Part model, mm, in its own coordinate system. Face numbers are marked on the shaded views. Give positions to 0.01 mm unless a question says otherwise; leave off trailing zeros. Order: outer loops, then holes, each group sorted by start corner. A loop starts at its lowest first (then second) coordinate and runs counter-clockwise, first axis right, second up. Notation, with made-up numbers: (56.25, 89.25) -> (87.25, 89.25) arc R22 ccw to (87.25, 118.25) -> close; hole circle Ø2 at (17.25, -30). An arc over 180 degrees is marked (long way). Write item = value, one per line. Start each with the question number.
(1) Flat gauge pins, fed straight in: pin 1 (3 mm diameter, centred on x = 4, z = 3.5, fed in from -Y); pin 2 (2 mm diameter, centred on y = -3, z = 7.5, fed in from -X); pin 3 (2 mm diameter, centred on x = 2, z = 4, fed in from -Y). Where does each tip first touch, or does it go through?
(2) Saw through at B-B, the plane x = 2.5. List the corners of the cut face in (y, z), then the cut area to 3 significant figures.
(3) Two-plate mould, pull along X, no slides. Class the marked faces 1, 2 and 3: pulls with the +X half, pulls with the -X half, needs draft (parallel to the pull), parting line crosses it, or undercut.
(4) Probe line 1 along Y through (x, z) = (0, 6.5); line 2 along Z through (x, y) = (0, 1.5); line 3 along X through (y, z) = (0.5, 4). List the from-to ranges inside material, lowest first. Write a range as from..to.
(5) Saw through at A-A, the plane y = 0. List the corners of the cut face in (x, z).
(6) Saw through at D-D, the plane y = -2. List the corners of the cut face in (x, z), then the cut area to 3 significant figures.
(7) Saw through at C-C, the plane z = 3. List the corners of the cut face in (x, y).
Autodesk Inventor part; units mm, degrees
ref_plane "YZ Plane" through (0, 0, 0) normal (1, 0, 0) x (0, 1, 0)
ref_plane "XZ Plane" through (0, 0, 0) normal (0, 1, 0) x (-1, 0, 0)
ref_plane "XY Plane" through (0, 0, 0) normal (0, 0, 1) x (1, 0, 0)
sketch "Sketch1" plane through (0, 0, 0) normal (0, 0, 1) x (1, 0, 0)
  line L0 (0, 8.8) -> (0, -6.6)
  line L1 (-6.6, 0) -> (8.8, 0)
  circle A0 centre (0, 0) radius 5.5
  dimension "d0" = 11
extrude "Extrusion1" add sketch "Sketch1" along normal blind 8.5
sketch "Sketch2" plane through (0, 0, 8.5) normal (0, 0, 1) x (1, 0, 0)
  circle A0 centre (0, 0) radius 5.5
  circle A1 centre (0, 0) radius 0.75
  dimension "d3" = 1.5
extrude "Extrusion2" cut sketch "Sketch2" against normal through all contours A1
sketch "Sketch3" plane through (0, 0, 8.5) normal (0, 0, 1) x (1, 0, 0)
  line L0 (-4.1622, 3.2044) -> (11.3317, 3.2044) construction
  line L1 (11.3317, 3.2044) -> (11.3317, -0.2956) construction
  line L2 (11.3317, -0.2956) -> (-4.1622, -0.2956) construction
  line L3 (-4.1622, -0.2956) -> (-4.1622, 3.2044) construction
  line L4 (-1.3375, -1.694) -> (1.5169, -1.694) construction
  line L5 (1.5169, -1.694) -> (1.5169, -4.135) construction
  line L6 (1.5169, -4.135) -> (-1.3375, -4.135) construction
  line L7 (-1.3375, -4.135) -> (-1.3375, -1.694) construction
  line L8 (-3.958, 3.2044) -> (-3.1577, 3.2044)
  spline S0 degree 5 poles (-3.1577, 3.2044) (-2.9199, 3.2044) (-2.6866, 3.1648) (-2.5022, 3.0398) (-2.3787, 2.8309) (-2.3787, 2.7014) knots 0 0 0 0 0 0 1 1 1 1 1 1
  spline S1 degree 3 poles (-2.3787, 2.7014) (-2.3787, 2.5611) (-2.5296, 2.3279) (-2.6592, 2.2684) knots 0 0 0 0 1 1 1 1
  spline S2 degree 3 poles (-2.6592, 2.2684) (-2.4763, 2.2151) (-2.2811, 1.959) (-2.2811, 1.7852) knots 0 0 0 0 1 1 1 1
  spline S3 degree 4 poles (-2.2811, 1.7852) (-2.2811, 1.648) (-2.4077, 1.3904) (-2.6287, 1.2364) (-2.7888, 1.2181) knots 0 0 0 0 0 1 1 1 1 1
  spline S4 degree 2 poles (-2.7888, 1.2181) (-2.8909, 1.2074) (-3.2766, 1.2044) knots 0 0 0 1 1 1
  line L9 (-3.2766, 1.2044) -> (-3.958, 1.2044)
  line L10 (-3.958, 1.2044) -> (-3.958, 3.2044)
  line L11 (-3.554, 2.0779) -> (-3.554, 1.5428)
  line L12 (-3.554, 1.5428) -> (-3.179, 1.5428)
  spline S5 degree 2 poles (-3.179, 1.5428) (-2.9595, 1.5428) (-2.9016, 1.555) knots 0 0 0 1 1 1
  spline S6 degree 3 poles (-2.9016, 1.555) (-2.8116, 1.5718) (-2.6973, 1.6983) (-2.6973, 1.805) knots 0 0 0 0 1 1 1 1
  spline S7 degree 4 poles (-2.6973, 1.805) (-2.6973, 1.8949) (-2.7842, 2.0199) (-2.9504, 2.0779) (-3.2263, 2.0779) knots 0 0 0 0 0 1 1 1 1 1
  line L13 (-3.2263, 2.0779) -> (-3.554, 2.0779)
  line L14 (-3.554, 2.8721) -> (-3.554, 2.4102)
  line L15 (-3.554, 2.4102) -> (-3.2888, 2.4102)
  spline S8 degree 2 poles (-3.2888, 2.4102) (-3.0525, 2.4102) (-2.9946, 2.4163) knots 0 0 0 1 1 1
  spline S9 degree 3 poles (-2.9946, 2.4163) (-2.8909, 2.43) (-2.772, 2.5474) (-2.772, 2.6449) knots 0 0 0 0 1 1 1 1
  spline S10 degree 3 poles (-2.772, 2.6449) (-2.772, 2.7379) (-2.8741, 2.8523) (-2.9763, 2.866) knots 0 0 0 0 1 1 1 1
  spline S11 degree 2 poles (-2.9763, 2.866) (-3.0357, 2.8721) (-3.3223, 2.8721) knots 0 0 0 1 1 1
  line L16 (-3.3223, 2.8721) -> (-3.554, 2.8721)
  line L17 (-1.9397, 1.2044) -> (-1.9397, 3.2044)
  line L18 (-1.9397, 3.2044) -> (-0.4565, 3.2044)
  line L19 (-0.4565, 3.2044) -> (-0.4565, 2.866)
  line L20 (-0.4565, 2.866) -> (-1.5357, 2.866)
  line L21 (-1.5357, 2.866) -> (-1.5357, 2.4224)
  line L22 (-1.5357, 2.4224) -> (-0.5311, 2.4224)
  line L23 (-0.5311, 2.4224) -> (-0.5311, 2.084)
  line L24 (-0.5311, 2.084) -> (-1.5357, 2.084)
  line L25 (-1.5357, 2.084) -> (-1.5357, 1.5428)
  line L26 (-1.5357, 1.5428) -> (-0.4183, 1.5428)
  line L27 (-0.4183, 1.5428) -> (-0.4183, 1.2044)
  line L28 (-0.4183, 1.2044) -> (-1.9397, 1.2044)
  line L29 (-0.2491, 1.2044) -> (-0.2491, 1.5687)
  line L30 (-0.2491, 1.5687) -> (0.8042, 2.866)
  line L31 (0.8042, 2.866) -> (-0.1302, 2.866)
  line L32 (-0.1302, 2.866) -> (-0.1302, 3.2044)
  line L33 (-0.1302, 3.2044) -> (1.3332, 3.2044)
  line L34 (1.3332, 3.2044) -> (1.3332, 2.8904)
  line L35 (1.3332, 2.8904) -> (0.2387, 1.5428)
  line L36 (0.2387, 1.5428) -> (1.3759, 1.5428)
  line L37 (1.3759, 1.5428) -> (1.3759, 1.2044)
  line L38 (1.3759, 1.2044) -> (-0.2491, 1.2044)
  line L39 (1.632, 1.2044) -> (1.632, 3.2044)
  line L40 (1.632, 3.2044) -> (3.1152, 3.2044)
  line L41 (3.1152, 3.2044) -> (3.1152, 2.866)
  line L42 (3.1152, 2.866) -> (2.0359, 2.866)
  line L43 (2.0359, 2.866) -> (2.0359, 2.4224)
  line L44 (2.0359, 2.4224) -> (3.0405, 2.4224)
  line L45 (3.0405, 2.4224) -> (3.0405, 2.084)
  line L46 (3.0405, 2.084) -> (2.0359, 2.084)
  line L47 (2.0359, 2.084) -> (2.0359, 1.5428)
  line L48 (2.0359, 1.5428) -> (3.1533, 1.5428)
  line L49 (3.1533, 1.5428) -> (3.1533, 1.2044)
  line L50 (3.1533, 1.2044) -> (1.632, 1.2044)
  line L51 (3.507, 1.2044) -> (3.507, 3.1876)
  line L52 (3.507, 3.1876) -> (3.9109, 3.1876)
  line L53 (3.9109, 3.1876) -> (3.9109, 1.5428)
  line L54 (3.9109, 1.5428) -> (4.9155, 1.5428)
  line L55 (4.9155, 1.5428) -> (4.9155, 1.2044)
  line L56 (4.9155, 1.2044) -> (3.507, 1.2044)
  line L57 (-0.2171, -4.135) -> (-0.2171, -3.2279)
  line L58 (-0.2171, -3.2279) -> (-1.1348, -3.2279)
  line L59 (-1.1348, -3.2279) -> (-1.1348, -2.601)
  line L60 (-1.1348, -2.601) -> (-0.2171, -2.601)
  line L61 (-0.2171, -2.601) -> (-0.2171, -1.694)
  line L62 (-0.2171, -1.694) -> (0.3938, -1.694)
  line L63 (0.3938, -1.694) -> (0.3938, -2.601)
  line L64 (0.3938, -2.601) -> (1.3142, -2.601)
  line L65 (1.3142, -2.601) -> (1.3142, -3.2279)
  line L66 (1.3142, -3.2279) -> (0.3938, -3.2279)
  line L67 (0.3938, -3.2279) -> (0.3938, -4.135)
  line L68 (0.3938, -4.135) -> (-0.2171, -4.135)
extrude "Extrusion3" cut sketch "Sketch3" against normal blind 0.05
properties part number "config - bezel"
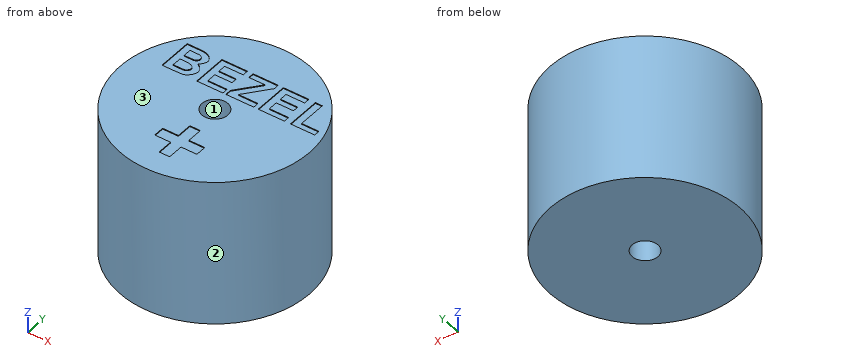
Results list:
q1.pin_1 = -4.9
q1.pin_2 = -5.12
q1.pin_3 = -5.41
q2.outline = (-4.9, 0) -> (4.9, 0) -> (4.9, 8.5) -> (3.2, 8.5) -> (3.2, 8.45) -> (2.87, 8.45) -> (2.87, 8.5) -> (2.42, 8.5) -> (2.42, 8.45) -> (2.08, 8.45) -> (2.08, 8.5) -> (1.54, 8.5) -> (1.54, 8.45) -> (1.2, 8.45) -> (1.2, 8.5) -> (-4.9, 8.5) -> close
q2.area = 83.2 mm^2
q3.face_1 = undercut
q3.face_2 = parting line crosses it
q3.face_3 = needs draft
q4.line_1 = -5.5..-0.75, 0.75..5.5
q4.line_2 = 0..8.45
q4.line_3 = -5.48..-0.56, 0.56..5.48
q5.outline = (-5.5, 0) -> (-0.75, 0) -> (-0.75, 8.5) -> (-5.5, 8.5) -> close; (0.75, 0) -> (5.5, 0) -> (5.5, 8.5) -> (0.75, 8.5) -> close
q6.outline = (-5.12, 0) -> (5.12, 0) -> (5.12, 8.5) -> (0.39, 8.5) -> (0.39, 8.45) -> (-0.22, 8.45) -> (-0.22, 8.5) -> (-5.12, 8.5) -> close
q6.area = 87.1 mm^2
q7.outline = circle Ø11 at (0, 0); hole circle Ø1.5 at (0, 0)
